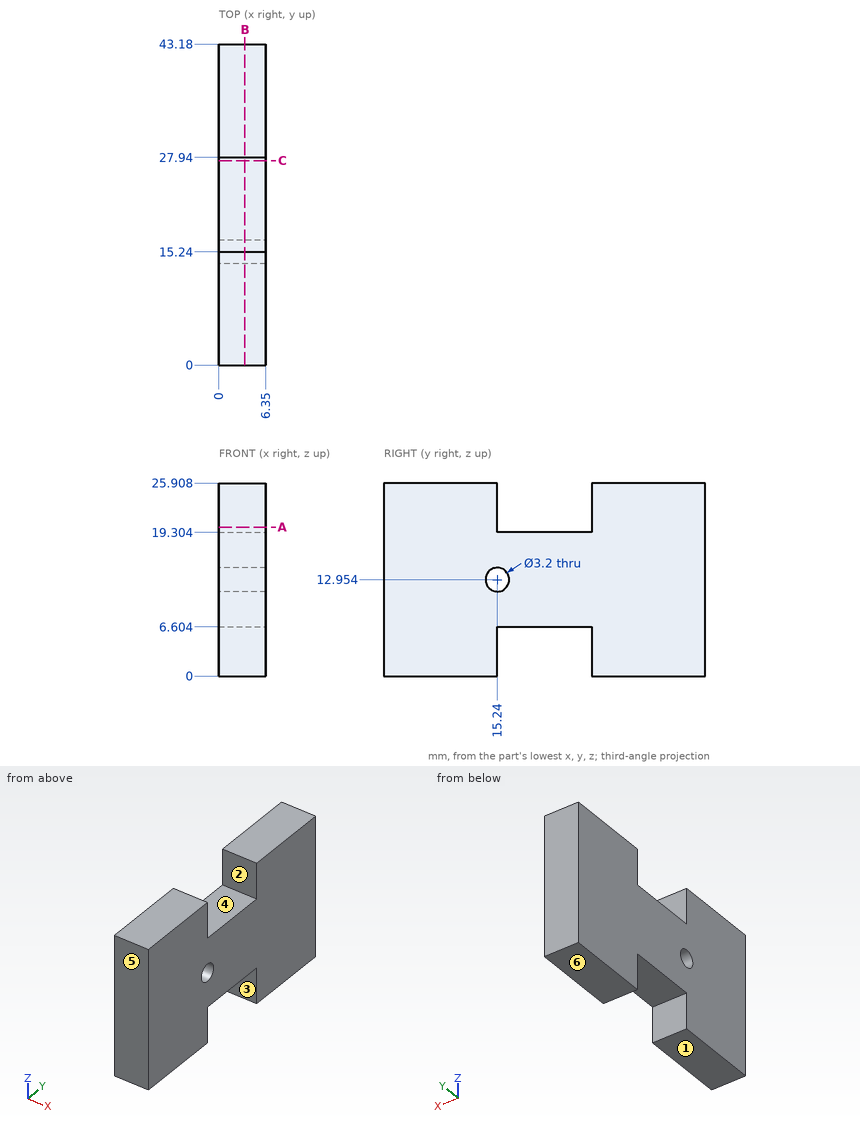
Verification items for this drawing (mm, ordinates from the low corner). A direction names the side the tool comes from. Round coordinates to 2 decimals unless told otherwise and drop trailing zeros. Write each loop counter-clockwise with the first axis right and the second up, starting at its lowest first coordinate (ties: lowest second). Pieces come first, ordered by that corner, then holes. Notation, with made-up numbers: (-12.75, 68) - (-4.75, 68) arc R30 ccw to (-4.75, 92) - close; hole circle Ø3 at (-12.5, 4). An arc over 180 degrees is marked (long way). One line per item, written item: value.
1. Cross-section at C-C on y = 27.5. Record the boundary of the cut face in (x, z).
The answers:
outline: (0, 6.6) - (6.35, 6.6) - (6.35, 19.3) - (0, 19.3) - close
2. Scan lines: L1, parallel to Y at x = 5.75, z = 3; L2, parallel to Z at x = 1, y = 18; L3, parallel to Y at x = 4.25, z = 13. Record each from-to range of solid material in increasing order.
The answers:
L1: y = 0 to 15.24, 27.94 to 43.18
L2: z = 6.6 to 19.3
L3: y = 0 to 13.64, 16.84 to 43.18
3. Mould release check, pull along Y, two halves, no side actions. Record for the marked faces 4, 5 and 6: released by +Y, released by -Y, zero draft, split by the parting line, or undercut.
The answers:
face 4: undercut
face 5: released by -Y
face 6: zero draft
4. Set-up check for the marked faces 1, 2 and 3: record each of +Z, -Z, +X, -X, +Y, -Y from which the full face is reachable in a straight line by a thin tool's end or side.
The answers:
face 1: -Z, +X, -X, +Y, -Y
face 2: +Z, +X, -X
face 3: -Z, +X, -X
5. Cross-section at A-A on z = 20. Record the boundary of the cut face in (x, y).
The answers:
outline: (0, 0) - (6.35, 0) - (6.35, 15.24) - (0, 15.24) - close; (0, 27.94) - (6.35, 27.94) - (6.35, 43.18) - (0, 43.18) - close
6. Cross-section at B-B on x = 3.5. Record the boundary of the cut face in (y, z), and give its area (3 significant figures).
The answers:
outline: (0, 0) - (15.24, 0) - (15.24, 6.6) - (27.94, 6.6) - (27.94, 0) - (43.18, 0) - (43.18, 25.91) - (27.94, 25.91) - (27.94, 19.3) - (15.24, 19.3) - (15.24, 25.91) - (0, 25.91) - close; hole circle Ø3.2 at (15.24, 12.95)
area: 943 mm^2
7. Depth check by flat-ended pin: pin 1 Ø1.9 at (x, y) = (4.5, 23.5) entering from +Z. Enter the tip coordinate at first touch or a pass-through.
The answers:
pin 1: stops at z = 19.3
